Here's the drawing with two shaded views (mm, measured from the low corner). I have some questions. A direction names the side the tool comes from. Round coordinates to 2 decimals unless told otherwise and drop trailing zeros. Loops run counter-clockwise (first coordinate to the right, second up) from the corner with the lowest first, then second, coordinate; pieces in that order, holes last. Notation, with made-up numbers: (-2.5, 85.5) - (33.5, 85.5) arc R26 ccw to (33.5, 116.5) - close; hole circle Ø11 at (15, 60). An arc over 180 degrees is marked (long way). Answer as CSV lines item,"result".
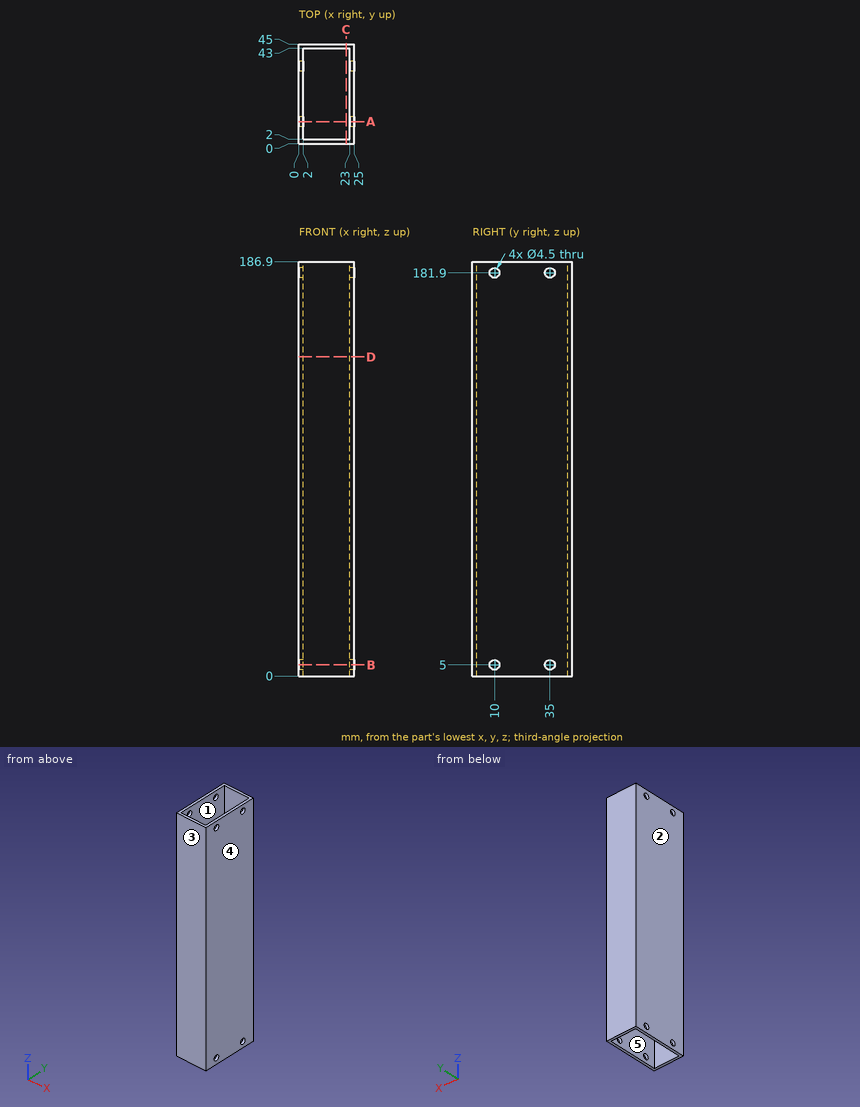
Q1. Imagine slicing it at B-B (z = 5). Write out the boundary of the cut face in (x, y).
Checks:
outline,"(0, 0) - (25, 0) - (25, 7.75) - (23, 7.75) - (23, 2) - (2, 2) - (2, 7.75) - (0, 7.75) - close; (0, 12.25) - (2, 12.25) - (2, 32.75) - (0, 32.75) - close; (0, 37.25) - (2, 37.25) - (2, 43) - (23, 43) - (23, 37.25) - (25, 37.25) - (25, 45) - (0, 45) - close; (23, 12.25) - (25, 12.25) - (25, 32.75) - (23, 32.75) - close"
Q2. Imagine slicing it at C-C (x = 21.25). Write out the boundary of the cut face in (y, z), then the cut area to 3 significant figures.
Checks:
outline,"(0, 0) - (2, 0) - (2, 186.9) - (0, 186.9) - close; (43, 0) - (45, 0) - (45, 186.9) - (43, 186.9) - close"
area,"748 mm²"
Q3. I'm going to push a flat-ended pin straight in: pin 1 Ø3.5 at (y, z) = (10, 5) entering from -X. Where does the tip first touch, or does it pass through?
Checks:
pin 1,"through"
Q4. We'd pull the mould along X, two halves only. Please class the marked faces 3, 4 and 5: pulls with the +X half, pulls with the -X half, needs draft (parallel to the pull), parting line crosses it, or undercut.
Checks:
face 3,"needs draft"
face 4,"pulls with the +X half"
face 5,"undercut"
Q5. On a 3-axis mill with a long thin cutter (end or side, diameter ignored), from which of +Z, -Z, +X, -X, +Y, -Y can I reach the whole of each face in a straight line? I mean the marked faces 1 and 2. Say none if no direction works.
Checks:
face 1,"+Z, -Z"
face 2,"+Z, -Z, -X, +Y, -Y"
Q6. Imagine slicing it at A-A (y = 10). Write out the boundary of the cut face in (x, z), then the cut area to 3 significant figures.
Checks:
outline,"(0, 0) - (2, 0) - (2, 2.75) - (0, 2.75) - close; (0, 7.25) - (2, 7.25) - (2, 179.65) - (0, 179.65) - close; (0, 184.15) - (2, 184.15) - (2, 186.9) - (0, 186.9) - close; (23, 0) - (25, 0) - (25, 2.75) - (23, 2.75) - close; (23, 7.25) - (25, 7.25) - (25, 179.65) - (23, 179.65) - close; (23, 184.15) - (25, 184.15) - (25, 186.9) - (23, 186.9) - close"
area,"712 mm²"
Q7. Imagine slicing it at D-D (z = 144). Write out the boundary of the cut face in (x, y).
Checks:
outline,"(0, 0) - (25, 0) - (25, 45) - (0, 45) - close; hole (2, 2) - (23, 2) - (23, 43) - (2, 43) - close"
Q8. If I drill on line 1 along Y through (x, z) = (23.6, 5); line 2 along X through (y, z) = (14, 140.5); line 3 along Y through (x, z) = (13, 141.5), over which ranges is the centre line in solid material (lowest first)? Write a range as [from, to].
Checks:
line 1,"[0, 7.75], [12.25, 32.75], [37.25, 45]"
line 2,"[0, 2], [23, 25]"
line 3,"[0, 2], [43, 45]"
